```python
from build123d import *

# Parameters (mm, degrees)
F0_R     = 2.5
F1_DEPTH = 750


with BuildPart() as f1:
    # F0 (on Right) → F1 (new body)
    with BuildSketch(Plane.YZ):
        Polygon((-22.87, 25.623863), (-15.373863, 33.12), (-16.88, 33.12), (-16.88, 34.626137), (-22.87, 28.636137), (-22.87, 34.25), (-25, 34.25), (-25, 15.75), (-22.87, 15.75), (-22.87, 21.363863), (-16.88, 15.373863), (-16.88, 16.88), (-15.373863, 16.88), (-22.87, 24.376137), align=None)
        Polygon((-8.12, 40.373863), (-8.12, 41.88), (-9.626137, 41.88), (-15.373863, 41.88), (-16.88, 41.88), (-16.88, 40.373863), (-16.88, 34.626137), (-16.88, 33.12), (-15.373863, 33.12), (-8.12, 33.12), align=None)
        with Locations((-12.5, 37.5)):
            Circle(F0_R, mode=Mode.SUBTRACT)
        Polygon((-16.88, 41.88), (-15.373863, 41.88), (-21.363863, 47.87), (-15.75, 47.87), (-15.75, 50), (-25, 50), (-25, 40.75), (-22.87, 40.75), (-22.87, 46.363863), (-16.88, 40.373863), align=None)
        Polygon((-9.626137, 41.88), (-8.12, 41.88), (-8.12, 40.373863), (-0.623863, 47.87), (0, 47.87), (0.623863, 47.87), (8.12, 40.373863), (8.12, 41.88), (9.626137, 41.88), (3.636137, 47.87), (9.25, 47.87), (9.25, 50), (0, 50), (-9.25, 50), (-9.25, 47.87), (-3.636137, 47.87), align=None)
        Polygon((8.12, 41.88), (8.12, 40.373863), (8.12, 33.12), (15.373863, 33.12), (16.88, 33.12), (16.88, 34.626137), (16.88, 40.373863), (16.88, 41.88), (15.373863, 41.88), (9.626137, 41.88), align=None)
        with Locations((12.5, 37.5)):
            Circle(F0_R, mode=Mode.SUBTRACT)
        Polygon((-0.623863, -47.87), (-8.12, -40.373863), (-8.12, -41.88), (-9.626137, -41.88), (-3.636137, -47.87), (-9.25, -47.87), (-9.25, -50), (0, -50), (9.25, -50), (9.25, -47.87), (3.636137, -47.87), (9.626137, -41.88), (8.12, -41.88), (8.12, -40.373863), (0.623863, -47.87), (0, -47.87), align=None)
        Polygon((15.373863, -8.12), (9.626137, -8.12), (8.12, -8.12), (8.12, -9.626137), (8.12, -16.88), (15.373863, -16.88), (16.88, -16.88), (16.88, -15.373863), (16.88, -9.626137), (16.88, -8.12), align=None)
        with Locations((12.5, -12.5)):
            Circle(F0_R, mode=Mode.SUBTRACT)
        Polygon((16.88, -16.88), (15.373863, -16.88), (22.87, -24.376137), (22.87, -25.623863), (15.373863, -33.12), (16.88, -33.12), (16.88, -34.626137), (22.87, -28.636137), (22.87, -34.25), (25, -34.25), (25, -15.75), (22.87, -15.75), (22.87, -21.363863), (16.88, -15.373863), align=None)
        Polygon((-8.12, 16.88), (-15.373863, 16.88), (-16.88, 16.88), (-16.88, 15.373863), (-16.88, 9.626137), (-16.88, 8.12), (-15.373863, 8.12), (-9.626137, 8.12), (-8.12, 8.12), (-8.12, 9.626137), align=None)
        with Locations((-12.5, 12.5)):
            Circle(F0_R, mode=Mode.SUBTRACT)
        Polygon((8.12, 16.88), (8.12, 9.626137), (8.12, 8.12), (9.626137, 8.12), (15.373863, 8.12), (16.88, 8.12), (16.88, 9.626137), (16.88, 15.373863), (16.88, 16.88), (15.373863, 16.88), align=None)
        with Locations((12.5, 12.5)):
            Circle(F0_R, mode=Mode.SUBTRACT)
        Polygon((-22.87, -24.376137), (-15.373863, -16.88), (-16.88, -16.88), (-16.88, -15.373863), (-22.87, -21.363863), (-22.87, -15.75), (-25, -15.75), (-25, -34.25), (-22.87, -34.25), (-22.87, -28.636137), (-16.88, -34.626137), (-16.88, -33.12), (-15.373863, -33.12), (-22.87, -25.623863), align=None)
        Polygon((-8.12, -8.12), (-9.626137, -8.12), (-15.373863, -8.12), (-16.88, -8.12), (-16.88, -9.626137), (-16.88, -15.373863), (-16.88, -16.88), (-15.373863, -16.88), (-8.12, -16.88), (-8.12, -9.626137), align=None)
        with Locations((-12.5, -12.5)):
            Circle(F0_R, mode=Mode.SUBTRACT)
        Polygon((16.88, 8.12), (15.373863, 8.12), (22.87, 0.623863), (22.87, 0), (22.87, -0.623863), (15.373863, -8.12), (16.88, -8.12), (16.88, -9.626137), (22.87, -3.636137), (22.87, -9.25), (25, -9.25), (25, 0), (25, 9.25), (22.87, 9.25), (22.87, 3.636137), (16.88, 9.626137), align=None)
        Polygon((16.88, 33.12), (15.373863, 33.12), (22.87, 25.623863), (22.87, 24.376137), (15.373863, 16.88), (16.88, 16.88), (16.88, 15.373863), (22.87, 21.363863), (22.87, 15.75), (25, 15.75), (25, 34.25), (22.87, 34.25), (22.87, 28.636137), (16.88, 34.626137), align=None)
        Polygon((-16.88, 8.12), (-16.88, 9.626137), (-22.87, 3.636137), (-22.87, 9.25), (-25, 9.25), (-25, 0), (-25, -9.25), (-22.87, -9.25), (-22.87, -3.636137), (-16.88, -9.626137), (-16.88, -8.12), (-15.373863, -8.12), (-22.87, -0.623863), (-22.87, 0), (-22.87, 0.623863), (-15.373863, 8.12), align=None)
        Polygon((21.363863, 47.87), (15.373863, 41.88), (16.88, 41.88), (16.88, 40.373863), (22.87, 46.363863), (22.87, 40.75), (25, 40.75), (25, 50), (15.75, 50), (15.75, 47.87), align=None)
        Polygon((22.87, -46.363863), (16.88, -40.373863), (16.88, -41.88), (15.373863, -41.88), (21.363863, -47.87), (15.75, -47.87), (15.75, -50), (25, -50), (25, -40.75), (22.87, -40.75), align=None)
        Polygon((-16.88, -41.88), (-16.88, -40.373863), (-22.87, -46.363863), (-22.87, -40.75), (-25, -40.75), (-25, -50), (-15.75, -50), (-15.75, -47.87), (-21.363863, -47.87), (-15.373863, -41.88), align=None)
        Polygon((16.88, -33.12), (15.373863, -33.12), (8.12, -33.12), (8.12, -40.373863), (8.12, -41.88), (9.626137, -41.88), (15.373863, -41.88), (16.88, -41.88), (16.88, -40.373863), (16.88, -34.626137), align=None)
        with Locations((12.5, -37.5)):
            Circle(F0_R, mode=Mode.SUBTRACT)
        Polygon((0, 1.506137), (-8.12, 9.626137), (-8.12, 8.12), (-9.626137, 8.12), (-1.506137, 0), (-9.626137, -8.12), (-8.12, -8.12), (-8.12, -9.626137), (0, -1.506137), (8.12, -9.626137), (8.12, -8.12), (9.626137, -8.12), (1.506137, 0), (9.626137, 8.12), (8.12, 8.12), (8.12, 9.626137), align=None)
        Polygon((-8.12, -33.12), (-15.373863, -33.12), (-16.88, -33.12), (-16.88, -34.626137), (-16.88, -40.373863), (-16.88, -41.88), (-15.373863, -41.88), (-9.626137, -41.88), (-8.12, -41.88), (-8.12, -40.373863), align=None)
        with Locations((-12.5, -37.5)):
            Circle(F0_R, mode=Mode.SUBTRACT)
    extrude(amount=F1_DEPTH)


solid = f1.part
```
Check sheet for the modelled part. Datum: model origin and axes. Units: mm. Round coordinates to 2 decimals unless told otherwise and drop trailing zeros. Write item = value, one per line. Start each with the question number.
1. Section check A-A, the plane x = 601.5. State how many separate pieces and enclosed holes the cut face has, then the cut area to 3 significant figures.
2. Scan lines: line 1 (Y direction, x = 239, z = -12); line 2 (Y direction, x = 162, z = 43); line 3 (Z direction, x = 81, y = -4). Record each from-to range of solid material in increasing order. Write a range as [from, to].
3. Gauge pin test, flat ends, axial feed: pin 1 (4.5 mm diameter, centred on x = 290.5, y = -12.5, fed in from +Z); pin 2 (2 mm diameter, centred on x = 385.5, y = -11, fed in from -Z). Record the tip position at first contact, or that the pin passes through.
Results found:
q1.separate_pieces = 1
q1.enclosed_holes = 12
q1.area = 1,390 mm^2
q2.line_1 = [-16.88, -14.95], [-10.05, -8.12], [8.12, 10.05], [14.95, 16.88]
q2.line_2 = [-25, -22.87], [-19.51, -16.49], [-8.51, -5.49], [5.49, 8.51], [16.49, 19.51], [22.87, 25]
q2.line_3 = [-50, -47.87], [-47.51, -44.49], [-5.51, -2.49], [2.49, 5.51], [44.49, 47.51], [47.87, 50]
q3.pin_1 = 41.88
q3.pin_2 = -41.88
